Check sheet for the drawn part. Datum: minimum x, y, z corner. Units: mm. A direction names the side the tool comes from. Coordinates: 2 decimals unless noted, no trailing zeros. Order: outer loops, then holes, each group sorted by start corner. A loop starts at its lowest first (then second) coordinate and runs counter-clockwise, first axis right, second up. Notation, with made-up numbers: (-30, 33.25) - (17, 33.25) arc R35 ccw to (17, 68.25) - close; hole circle Ø2 at (29, 26). An arc over 180 degrees is marked (long way). One line per item, written item: value. Start each with the question number.
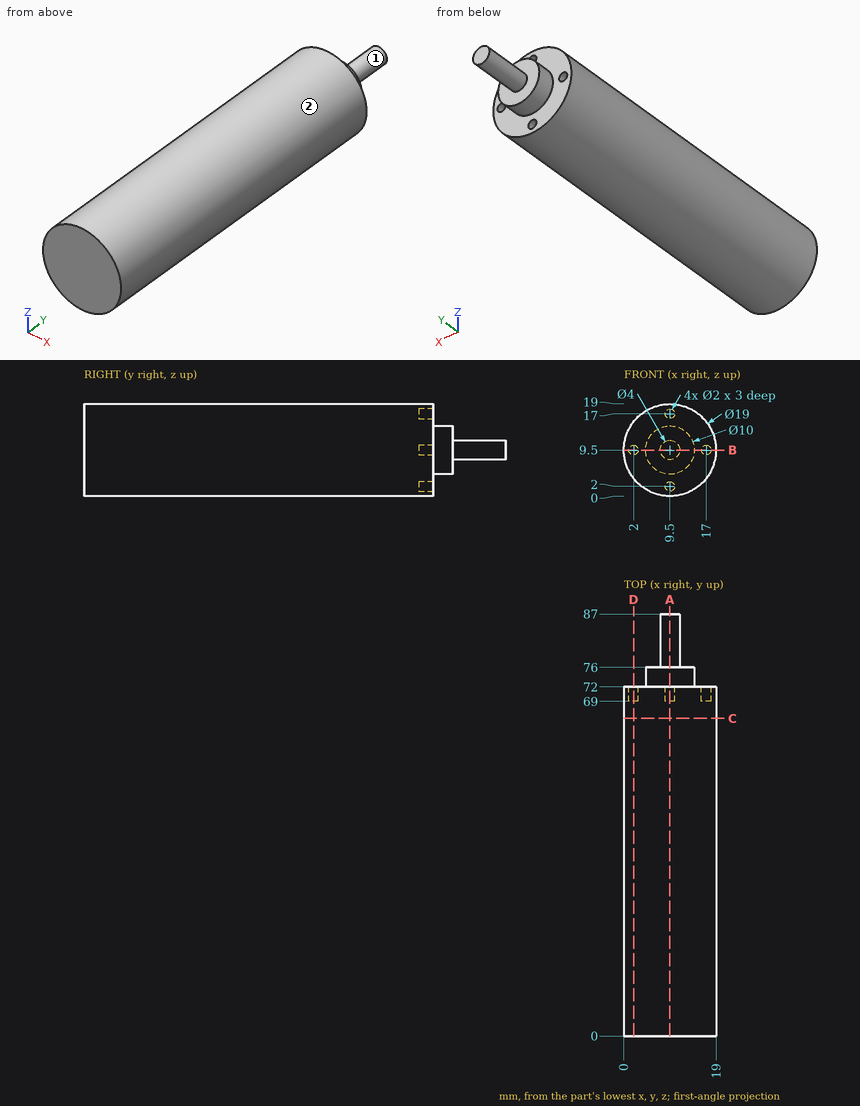
Q1. Cross-section at C-C, the plane y = 65.5. Enter the section's corners in (x, z), and give its area (3 significant figures).
Q2. Set-up check for the marked faces 1 and 2: record each of +Z, -Z, +X, -X, +Y, -Y from which the full face is reachable in a straight line by a thin tool's end or side.
Q3. Gauge pin test, flat ends, axial feed: P1, Ø4, axis at y = 9, z = 2, coming from the +X side; P2, Ø6, axis at x = 4.5, y = 47.5, coming from the -Z side; P3, Ø6, axis at x = 3, z = 6.5, coming from the +Y side. Record the tip position at first contact, or that the pin passes through.
Q4. Cross-section at B-B, the plane z = 9.5. Enter the section's corners in (x, y), and give its area (3 significant figures).
Q5. Material ranges on probe 1 along X at (y, z) = (70.3, 9.5); probe 2 along Y at (x, z) = (9.25, 2.5); probe 3 along Y at (x, z) = (15.25, 4), recorded low to high.
Q6. Cross-section at D-D, the plane x = 2. Enter the section's corners in (y, z), and give its area (3 significant figures).
Q7. Cross-section at A-A, the plane x = 9.5. Enter the section's corners in (y, z), and give its area (3 significant figures).
Check result:
1. outline: circle Ø19 at (9.5, 9.5)
1. area: 284 mm2
2. face 1: +Y
2. face 2: +Y, -Y
3. P1: stops at x = 17.25
3. P2: stops at z = 0.21
3. P3: stops at y = 76
4. outline: (0, 0) - (19, 0) - (19, 72) - (18, 72) - (18, 69) - (16, 69) - (16, 72) - (14.5, 72) - (14.5, 76) - (11.5, 76) - (11.5, 87) - (7.5, 87) - (7.5, 76) - (4.5, 76) - (4.5, 72) - (3, 72) - (3, 69) - (1, 69) - (1, 72) - (0, 72) - close
4. area: 1,440 mm2
5. probe 1: x = 0 to 1, 3 to 16, 18 to 19
5. probe 2: y = 0 to 69
5. probe 3: y = 0 to 72
6. outline: (0, 3.67) - (72, 3.67) - (72, 8.5) - (69, 8.5) - (69, 10.5) - (72, 10.5) - (72, 15.33) - (0, 15.33) - close
6. area: 834 mm2
7. outline: (0, 0) - (72, 0) - (72, 1) - (69, 1) - (69, 3) - (72, 3) - (72, 4.5) - (76, 4.5) - (76, 7.5) - (87, 7.5) - (87, 11.5) - (76, 11.5) - (76, 14.5) - (72, 14.5) - (72, 16) - (69, 16) - (69, 18) - (72, 18) - (72, 19) - (0, 19) - close
7. area: 1,440 mm2
